```python
from build123d import *

# Parameters (mm, degrees)
EXTRUDE_1_DEPTH     = 29
CUT_EXTRUDE_1_DEPTH = 29
CUT_EXTRUDE_2_DEPTH = 1
FILLET_1_R          = 0.5
EXTRUDE_2_DEPTH     = 1
SKETCH_7_R          = 2.75
SKETCH_7_R_2        = 1
EXTRUDE_5_DEPTH     = 22
CUT_EXTRUDE_START   = 19
SKETCH_8_R          = 6.25
CUT_EXTRUDE_4_DEPTH = 19
SKETCH_9_R          = 1
CUT_EXTRUDE_5_DEPTH = 18
SKETCH_10_R         = 1
CUT_EXTRUDE_6_DEPTH = 26


with BuildPart() as part:
    # 草图1 → 旋转1 (revolve)
    with BuildSketch(Plane.XY, mode=Mode.PRIVATE) as revolve_1_sk:
        Polygon((4, 0), (4, -3), (3.5, -3), (3.5, -6), (6, -6), (6, -9.5), (6.25, -9.5), (6.25, -16), (8, -16), (8, -4), (6, -4), (6, 0), align=None)
    revolve(revolve_1_sk.sketch.rotate(Axis((0, 0, 0), (0, -1, 0)), 180), axis=Axis((0, 0, 0), (0, -1, 0)))

    # 草图2 → 凸台-拉伸1 (add)
    with BuildSketch(Plane(origin=(0, -4, 0), x_dir=(1, 0, 0), z_dir=(0, 1, 0))):
        with BuildLine():
            Line((7.745966692, 2), (32, 2))
            Line((32, 2), (32, -2))
            Line((32, -2), (7.745966692, -2))
            ThreePointArc((7.745966692, -2), (8, 0), (7.745966692, 2))
        make_face()
    extrude(amount=-EXTRUDE_1_DEPTH)

    # 草图3 → 切除-拉伸1 (cut)
    with BuildSketch(Plane(origin=(0, 0, -12), x_dir=(-1, 0, 0), z_dir=(0, 0, -1))):
        with BuildLine():
            Line((8, -10), (1.860452447, -14.853447831))
            ThreePointArc((1.860452447, -14.853447831), (0.600535009, -15.439278432), (-0.788203157, -15.394604599))
            Line((-0.788203157, -15.394604599), (-7.745966692, -13.5))
            ThreePointArc((-7.745966692, -13.5), (-9.489135576, -13.468262993), (-11.037904709, -14.26886225))
            Line((-11.037904709, -14.26886225), (-20.611161345, -22.746001069))
            ThreePointArc((-20.611161345, -22.746001069), (-21.536515916, -23.305174077), (-22.6, -23.5))
            Line((-22.6, -23.5), (-26, -23.5))
            ThreePointArc((-26, -23.5), (-29, -20.5), (-26, -17.5))
            Line((-26, -17.5), (-24.491554542, -17.5))
            Line((-24.491554542, -17.5), (-9.245966692, -4))
            Line((-9.245966692, -4), (-32, -4))
            Line((-32, -4), (-32, -33))
            Line((-32, -33), (-7.745966692, -33))
            Line((-7.745966692, -33), (-7.745966692, -16))
            Line((-7.745966692, -16), (8, -16))
            Line((8, -16), (8, -10))
        make_face()
    extrude(amount=-CUT_EXTRUDE_1_DEPTH, mode=Mode.SUBTRACT)

    # 草图4 → 切除-拉伸2 (cut)
    with BuildSketch(Plane(origin=(0, 0, -2), x_dir=(-1, 0, 0), z_dir=(0, 0, -1))):
        with BuildLine():
            Line((-19.26013767, -19.746461933), (-21.7793333, -16.901527245))
            Line((-21.7793333, -16.901527245), (-8.595436654, -5.227159128))
            ThreePointArc((-8.595436654, -5.227159128), (-8.047086067, -5.143800877), (-7.745966692, -5.609594916))
            Line((-7.745966692, -5.609594916), (-7.745966692, -9.550639395))
            Line((-7.745966692, -9.550639395), (-19.26013767, -19.746461933))
        make_face()
    cut_extrude_2 = extrude(amount=-CUT_EXTRUDE_2_DEPTH, mode=Mode.SUBTRACT)

    # 圆角1
    fillet_1_edges = [part.edges().sort_by_distance(p)[0] for p in [
        (19.26013767, -19.746461933, -1.5),
        (21.7793333, -16.901527245, -1.5),
    ]]
    fillet(fillet_1_edges, radius=FILLET_1_R)

    # 草图5 → 凸台-拉伸2 (add)
    with BuildSketch(Plane(origin=(0, 0, -2), x_dir=(-1, 0, 0), z_dir=(0, 0, -1))):
        with BuildLine():
            Line((-22.6, -23), (-26, -23))
            ThreePointArc((-26, -23), (-28.5, -20.5), (-26, -18))
            Line((-26, -18), (-22.6, -18))
            ThreePointArc((-22.6, -18), (-20.1, -20.5), (-22.6, -23))
        make_face()
    extrude_2 = extrude(amount=EXTRUDE_2_DEPTH)

    # 镜向1: 切除-拉伸2, 凸台-拉伸2 across plane
    add(cut_extrude_2.mirror(Plane(origin=(0, 0, 0), x_dir=(1, 0, 0), z_dir=(0, 0, -1))), mode=Mode.SUBTRACT)
    add(extrude_2.mirror(Plane(origin=(0, 0, 0), x_dir=(1, 0, 0), z_dir=(0, 0, -1))))

    # 草图7 → 凸台-拉伸5 (add)
    with BuildSketch(Plane(origin=(0, 0, -11), x_dir=(-1, 0, 0), z_dir=(0, 0, -1))):
        with Locations((0, -12.45)):
            Circle(SKETCH_7_R)
        with Locations((0, -12.45)):
            Circle(SKETCH_7_R_2, mode=Mode.SUBTRACT)
    extrude(amount=-EXTRUDE_5_DEPTH)

    # 草图8 → 切除-拉伸4 (cut)
    with BuildSketch(Plane.XZ.offset(9.5).offset(CUT_EXTRUDE_START)):
        with Locations(Location((0, 0, 0), (0, 0, 180))):
            Circle(SKETCH_8_R)
    extrude(amount=-CUT_EXTRUDE_4_DEPTH, mode=Mode.SUBTRACT)

    # 草图9 → 切除-拉伸5 (cut)
    with BuildSketch(Plane(origin=(0, 0, -3), x_dir=(-1, 0, 0), z_dir=(0, 0, -1))):
        with Locations((-27, -20.45)):
            Circle(SKETCH_9_R)
        with Locations((-23.6, -20.45)):
            Circle(SKETCH_9_R)
    extrude(amount=-CUT_EXTRUDE_5_DEPTH, mode=Mode.SUBTRACT)

    # 草图10 → 切除-拉伸6 (cut)
    with BuildSketch(Plane(origin=(0, 0, -11), x_dir=(-1, 0, 0), z_dir=(0, 0, -1))):
        with Locations((0, -12.45)):
            Circle(SKETCH_10_R)
    extrude(amount=-CUT_EXTRUDE_6_DEPTH, mode=Mode.SUBTRACT)


solid = part.part
```
CAD build for the part. Positions are in the model's coordinates, mm. A direction names the side the tool comes from. Round coordinates to 2 decimals unless told otherwise and drop trailing zeros. Order: outer loops, then holes, each group sorted by start corner. A loop starts at its lowest first (then second) coordinate and runs counter-clockwise, first axis right, second up.
Item 1: Mould opens along X. For faces 1 (the face through (16.975, -10.844, -0.028)), 2 (the face through (25, -20, 3)), 3 (the face through (0.867, -1.521, 3.905)) say: pulls with the +X half, pulls with the -X half, needs draft (parallel to the pull), parting line crosses it, or undercut.
Item 2: Saw through at C-C on z = 0. State how many separate pieces and enclosed holes the cut face has, then the cut area to 3 significant figures.
Item 3: Probe line 1 along Z through (x, y) = (0, -9); line 2 along Y through (x, z) = (0, 8.7); line 3 along Z through (x, y) = (0, -4.7). List the from-to ranges inside material, lowest first.
Item 4: Tool access for faces 4 (the face through (-5.723, -1.972, -1.802)), 5 (the face through (14, -12, 1)), 6 (the face through (24.3, -18, 2.5)), 7 (the face through (28.5, -20.6, 2.5)): list every direction of +Z, -Z, +X, -X, +Y, -Y with a clear straight run to the whole face (end or side of a thin tool).
Item 5: Pin check, flat tips, straight feed: pin 1 (1.1 mm diameter, centred on y = -7, z = 1.5, fed in from +X) (3 decimals); pin 2 (0.8 mm diameter, centred on x = 25, z = -2.5, fed in from +Y); pin 3 (5.5 mm diameter, centred on x = 24.5, y = -21, fed in from +Z); pin 4 (1.6 mm diameter, centred on x = 23.6, y = -20.45, fed in from +Z). Stop position of each tip, or through.
Item 6: Saw through at B-B on y = -20.45. Write the cut outline in (x, z), then the cut area to 3 significant figures.
Item 7: Saw through at D-D on z = -9.5. Write the cut outline in (x, y), then the cut area to 3 significant figures.
Reported:
1. face 1: pulls with the +X half
1. face 2: needs draft
1. face 3: undercut
2. separate pieces: 2
2. enclosed holes: 2
2. area: 216 mm2
3. line 1: z = -8 to -6, 6 to 8
3. line 2: y = -15.2 to -13.45, -11.45 to -9.7
3. line 3: z = -8 to -3.5, 3.5 to 8
4. face 4: +Y
4. face 5: +Z
4. face 6: +Z, +X, -X, +Y
4. face 7: +Z, +X
5. pin 1: stops at x = 13.255
5. pin 2: stops at y = -18
5. pin 3: stops at z = 3
5. pin 4: passes through
6. outline: (18.02, -2) - (20.1, -2) - (20.1, -3) - (22.6, -3) - (22.6, 3) - (20.1, 3) - (20.1, 2) - (18.02, 2) - close; (24.6, -3) - (26, -3) - (26, 3) - (24.6, 3) - close; (28, -3) - (28.5, -3) - (28.5, -2) - (29, -2) - (29, 2) - (28.5, 2) - (28.5, 3) - (28, 3) - close
6. area: 36.7 mm2
7. outline: circle Ø5.5 at (0, -12.45); hole circle Ø2 at (0, -12.45)
7. area: 20.6 mm2
